```python
from build123d import *

# Parameters (mm, degrees)
F0_W     = 700
F0_H     = 400
F1_DEPTH = 5
F2_W     = 15
F2_H     = 200
F2_H_2   = 150
F3_DEPTH = 25


with BuildPart() as f1:
    # F0 (on Top) → F1 (new body)
    with BuildSketch(Plane.XY):
        Rectangle(F0_W, F0_H)
    extrude(amount=F1_DEPTH)

    # F2 (on face) → F3 (cut)
    with BuildSketch(Plane(origin=(0, 0, 0), x_dir=(1, 0, 0), z_dir=(0, 0, -1))):
        with Locations((187.5, 0)):
            Rectangle(F2_W, F2_H)
        with Locations((-107.5, -11.036794)):
            Rectangle(F2_W, F2_H_2)
    extrude(amount=-F3_DEPTH, mode=Mode.SUBTRACT)


solid = f1.part
```
Work out the finished part from the listing and answer in its coordinate system (mm). Give positions to 0.01 mm unless a question says otherwise; leave off trailing zeros. Order: outer loops, then holes, each group sorted by start corner. A loop starts at its lowest first (then second) coordinate and runs counter-clockwise, first axis right, second up. Notation, with made-up numbers: (40, 14.5) -> (89, 14.5) arc R22 ccw to (89, 46.5) -> close; hole circle Ø4 at (74.25, 3). An arc over 180 degrees is marked (long way). Answer as CSV lines item,"result". Start each with the question number.
(1) Section B-B, the plane y = -75 is taken. Write down the section's boundary in (x, z).
(2) Consider line 1 along X through (y, z) = (76, 1.8); line 2 along X through (y, z) = (-97.5, 0.45); line 3 along Y through (x, z) = (180.5, 2.95). Determine where each line is inside the solid, lowest interval first.
(3) Section C-C, the plane z = 3.65 is taken. Write down the section's boundary in (x, y).
(4) Section A-A, the plane y = -29 is taken. Write down the section's boundary in (x, z), plus the area to 3 significant figures.
Entries:
1,outline,"(-350, 0) -> (180, 0) -> (180, 5) -> (-350, 5) -> close; (195, 0) -> (350, 0) -> (350, 5) -> (195, 5) -> close"
2,line 1,"-350 to -115, -100 to 180, 195 to 350"
2,line 2,"-350 to 180, 195 to 350"
2,line 3,"-200 to -100, 100 to 200"
3,outline,"(-350, -200) -> (350, -200) -> (350, 200) -> (-350, 200) -> close; hole (-115, -63.96) -> (-100, -63.96) -> (-100, 86.04) -> (-115, 86.04) -> close; hole (180, -100) -> (195, -100) -> (195, 100) -> (180, 100) -> close"
4,outline,"(-350, 0) -> (-115, 0) -> (-115, 5) -> (-350, 5) -> close; (-100, 0) -> (180, 0) -> (180, 5) -> (-100, 5) -> close; (195, 0) -> (350, 0) -> (350, 5) -> (195, 5) -> close"
4,area,"3,350 mm²"
